Build history of the part. All positions in model axes, mm. A direction names the side the tool comes from. Round coordinates to 2 decimals unless told otherwise and drop trailing zeros. Loops run counter-clockwise (first coordinate to the right, second up) from the corner with the lowest first, then second, coordinate; pieces in that order, holes last. Notation, with made-up numbers: M -35,25 L -13,25 A27 cw -13,50 Z; hole C -13.75,75 d10. An arc over 180 degrees is marked long. Write each question's results on one line, items separated by ' | '. Start each with the question number.
```python
from build123d import *

# Parameters (mm, degrees)
SKETCH1_W           = 76.2
SKETCH1_H           = 25.4
SKETCH1_W_2         = 70.104
SKETCH1_H_2         = 19.304
BOSS_EXTRUDE1_DEPTH = 280
CUT_EXTRUDE1_START  = -34.530327
SKETCH3_W           = 25.4
SKETCH3_H           = 76.2
CUT_EXTRUDE1_DEPTH  = 72.630327
SKETCH5_W           = 76.2
SKETCH5_H           = 25.4
SKETCH5_W_2         = 70.104
SKETCH5_H_2         = 19.304
BOSS_EXTRUDE2_DEPTH = 38.1


with BuildPart() as part:
    # Sketch1 → Boss-Extrude1 (new body)
    with BuildSketch(Plane(origin=(0, 0, 0), x_dir=(1, 0, 0), z_dir=(0, 1, 0))):
        Rectangle(SKETCH1_W, SKETCH1_H)
        Rectangle(SKETCH1_W_2, SKETCH1_H_2, mode=Mode.SUBTRACT)
    extrude(amount=BOSS_EXTRUDE1_DEPTH)

    # Sketch3 → Cut-Extrude1 (cut)
    with BuildSketch(Plane(origin=(0, 0, 0), x_dir=(0, 0, -1), z_dir=(0.906307787, 0.422618262, 0)).offset(CUT_EXTRUDE1_START)):
        Rectangle(SKETCH3_W, SKETCH3_H)
    extrude(amount=CUT_EXTRUDE1_DEPTH, mode=Mode.SUBTRACT)

    # Sketch5 → Boss-Extrude2 (add)
    with BuildSketch(Plane(origin=(0, 280, 0), x_dir=(1, 0, 0), z_dir=(0, 1, 0))):
        Rectangle(SKETCH5_W, SKETCH5_H)
        Rectangle(SKETCH5_W_2, SKETCH5_H_2, mode=Mode.SUBTRACT)
    extrude(amount=BOSS_EXTRUDE2_DEPTH)


solid = part.part
```
Item 1: Mould opens along Z. For faces 1 (the flat face through (0, 164, 9.652)), 2 (the flat face through (-3, 318.1, 10)), 3 (the flat face through (-1, 161, -12.7)) say: released by +Z, released by -Z, zero draft, split by the parting line, or undercut.
Item 2: Drill centre lines: line 1 along X through (y, z) = (211, -5.5); line 2 along Z through (x, y) = (25.5, 224.5); line 3 along X through (y, z) = (24, -2). Where is each one in solid material? Low to high. Write a range as [from, to].
Item 3: Tool access for faces 4 (the flat face through (0, 164, -9.652)), 5 (the flat face through (38.1, 161, 0)), 6 (the flat face through (-16.25, 34.46, 10.41)): list every direction of +Z, -Z, +X, -X, +Y, -Y with a clear straight run to the whole face (end or side of a thin tool).
Item 4: Saw through at C-C, the plane x = 30.5. Give the cut face in (y, z).
Item 5: Saw through at B-B, the plane z = 6.5. Give the cut face in (x, y).
Item 6: Saw through at A-A, the plane y = 291. Give the cut face in (x, z).
Working result:
1) face 1: undercut | face 2: zero draft | face 3: released by -Z
2) line 1: x = [-38.1, -35.05], [35.05, 38.1] | line 2: z = [-12.7, -9.65], [9.65, 12.7] | line 3: x = [35.05, 38.1]
3) face 4: +Y, -Y | face 5: +Z, -Z, +X, +Y, -Y | face 6: +Z, -Z, -Y
4) outline: M 24.74,-12.7 L 318.1,-12.7 L 318.1,-9.65 L 24.74,-9.65 Z; M 24.74,9.65 L 318.1,9.65 L 318.1,12.7 L 24.74,12.7 Z
5) outline: M -38.1,24.27 L -35.05,25.69 L -35.05,318.1 L -38.1,318.1 Z; M 35.05,14.98 L 38.1,8.45 L 38.1,318.1 L 35.05,318.1 Z
6) outline: M -38.1,-12.7 L 38.1,-12.7 L 38.1,12.7 L -38.1,12.7 Z; hole M -35.05,-9.65 L 35.05,-9.65 L 35.05,9.65 L -35.05,9.65 Z
